```python
from build123d import *

# Parameters (mm, degrees)
F2_SIZE = 0.5
F3_SIZE = 0.4
F4_SIZE = 0.3


with BuildPart() as f1:
    # F0 (on Front) → F1 (revolve)
    with BuildSketch(Plane.XZ):
        Polygon((2.5, 0), (7.5, 0), (7.5, 1), (6.5, 1), (6.5, 4), (2.5, 4), align=None)
    revolve(axis=Axis((0, 0, 10.44), (0, 0, 1)))

    # F2
    f2_edges = [f1.edges().sort_by_distance(p)[0] for p in [
        (-6.5, 0, 4),
    ]]
    chamfer(f2_edges, length=F2_SIZE)

    # F3
    f3_edges = [f1.edges().sort_by_distance(p)[0] for p in [
        (-7.5, 0, 0),
    ]]
    chamfer(f3_edges, length=F3_SIZE)

    # F4
    f4_edges = [f1.edges().sort_by_distance(p)[0] for p in [
        (-2.5, 0, 0),
        (-2.5, 0, 4),
    ]]
    chamfer(f4_edges, length=F4_SIZE)


solid = f1.part
```
Check sheet for the modelled part. Datum: model origin and axes. Units: mm. A direction names the side the tool comes from. Give positions to 0.01 mm unless a question says otherwise; leave off trailing zeros. Write each loop counter-clockwise with the first axis right and the second up, starting at its lowest first coordinate (ties: lowest second). Pieces come first, ordered by that corner, then holes. Notation, with made-up numbers: (22.25, 27) -> (40.25, 27) arc R18 cw to (40.25, 42) -> close; hole circle Ø7 at (69, 89). An arc over 180 degrees is marked (long way). Use CSV: the item, a comma, the result in double quotes. Start each with the question number.
Q1. Depth check by flat-ended pin: P1, Ø2, axis at x = -5.5, z = 1, coming from the +Y side. Enter the tip coordinate at first touch or a pass-through.
Q2. Release check for a two-part mould opening along Y. For faces 1 (the cylindrical face through (-0.54, -2.44, 1.98)), 2 (the flat face through (0, -3, 0)), 3 (the cylindrical face through (-7.493, 0.33, 0.704)) record: +Y half, -Y half, draft (parallel to the pull), parting line (faces both ways), or undercut.
Q3. Tool access check on faces 4 (the cylindrical face through (-5.158, -3.955, 2.268)), 5 (the flat face through (3, -1, 4)). Record the directions out of +Z, -Z, +X, -X, +Y, -Y that give a thin tool (end or side, any length) a straight path to the whole face; none if there is none.
Q4. Cross-section at A-A on y = 0. Enter the section's corners in (x, z).
Q5. Scan lines: line 1 along Y through (x, z) = (0, 1.7); line 2 along Y through (x, z) = (-2.25, 0.35); line 3 along X through (y, z) = (6, 1.5). Record each from-to range of solid material in increasing order.
Q6. Cross-section at C-C on z = 1.75. Enter the section's corners in (x, y), and give its area (3 significant figures).
Working result:
1,P1,"stops at y = 6"
2,face 1,"undercut"
2,face 2,"draft"
2,face 3,"parting line"
3,face 4,"+Z"
3,face 5,"+Z, +X, -X, +Y, -Y"
4,outline,"(-7.5, 0.4) -> (-7.1, 0) -> (-2.8, 0) -> (-2.5, 0.3) -> (-2.5, 3.7) -> (-2.8, 4) -> (-6, 4) -> (-6.5, 3.5) -> (-6.5, 1) -> (-7.5, 1) -> close; (2.5, 0.3) -> (2.8, 0) -> (7.1, 0) -> (7.5, 0.4) -> (7.5, 1) -> (6.5, 1) -> (6.5, 3.5) -> (6, 4) -> (2.8, 4) -> (2.5, 3.7) -> close"
5,line 1,"y = -6.5 to -2.5, 2.5 to 6.5"
5,line 2,"y = -7.1 to -1.09, 1.09 to 7.1"
5,line 3,"x = -2.5 to 2.5"
6,outline,"circle Ø13 at (0, 0); hole circle Ø5 at (0, 0)"
6,area,"113 mm^2"
